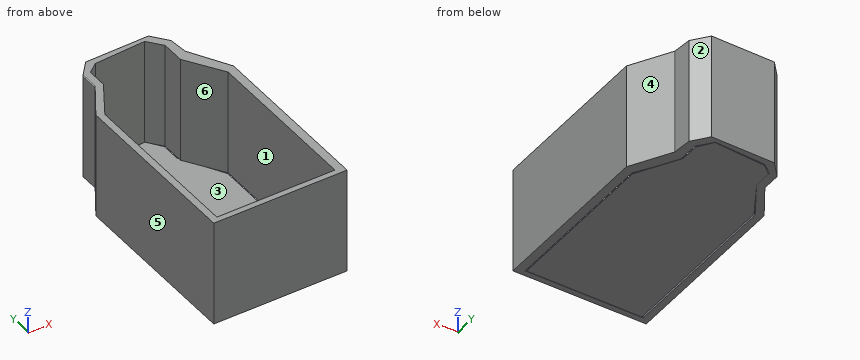
from build123d import *

# Parameters (mm, degrees)
F1_DEPTH = 53.34
F3_DEPTH = 0.254
F4_R     = 0.427399


with BuildPart() as f1:
    # F0 (on Top) → F1 (new body)
    with BuildSketch(Plane.XY):
        Polygon((-29.670693, 53.525094), (-40.17527, 37.058461), (-40.17527, -53.224109), (27.1108, -53.224109), (27.1108, 33.651568), (15.754499, 53.525094), (14.902776, 62.894039), (8.656814, 70.843451), (-23.42473, 70.275635), (-29.670693, 62.894039), align=None)
        Polygon((-25.695989, 63.177943), (-20.585654, 67.152657), (5.249925, 68.572186), (10.928073, 61.474502), (10.928073, 49.834296), (22.85219, 31.380311), (22.85219, -50.385039), (-36.768381, -50.385039), (-36.768381, 35.355017), (-25.695989, 53.241186), align=None, mode=Mode.SUBTRACT)
    extrude(amount=F1_DEPTH)

    # F2 (on Top) → F3 (join)
    with BuildSketch(Plane.XY):
        Polygon((-18.457072, 66.836618), (-20.728331, 66.836618), (-25.554758, 62.578008), (-25.554758, 53.492971), (-35.775427, 35.890706), (-35.775427, -49.84935), (22.425605, -49.84935), (22.425605, 31.064278), (10.501488, 51.789522), (10.501488, 61.442375), (5.391155, 68.540059), align=None)
    extrude(amount=-F3_DEPTH)

    # F4
    f4_edges = [f1.edges().sort_by_distance(p)[0] for p in [
        (-36.768381, 35.355017, 26.67),
        (-29.670693, 58.209566, 53.34),
        (15.754499, 53.525094, 26.67),
    ]]
    fillet(f4_edges, radius=F4_R)


solid = f1.part
Read the model definition and answer for the solid it produces. Units are mm, in the model's axes. Face numbers are marked on the shaded views. A direction names the side the tool comes from. Give positions to 0.01 mm unless a question says otherwise; leave off trailing zeros. Loops run counter-clockwise (first coordinate to the right, second up) from the corner with the lowest first, then second, coordinate; pieces in that order, holes last. Notation, with made-up numbers: (57, 14) -> (113, 14) arc R22 cw to (113, 52) -> close; hole circle Ø11 at (-17.5, -39.5). An arc over 180 degrees is marked (long way). Answer as CSV lines item,"result".
Item 1: Determine the mould class of the marked faces 4, 5 and 6 for opening direction X: +X half, -X half, draft (parallel to the pull), parting line (faces both ways), or undercut.
Returned:
face 4,"+X half"
face 5,"-X half"
face 6,"undercut"
Item 2: Each of these flat-tipped pins is pushed along its axis until it touches: pin 1 (2 mm diameter, centred on x = 4.5, y = 57.5, fed in from +Z); pin 2 (1.5 mm diameter, centred on y = 55.5, z = 6.5, fed in from +X); pin 3 (10 mm diameter, centred on x = 1, z = 5.5, fed in from +Y). Where does it stop, or does it pass through?
Returned:
pin 1,"stops at z = 0"
pin 2,"stops at x = 15.64"
pin 3,"stops at y = 70.8"
Item 3: Find section D-D on y = 48.5. Give the vertices of the cut face in (x, z), plus the area to 3 significant figures.
Returned:
outline,"(-32.88, 0) -> (-28.63, 0) -> (-28.63, 53.34) -> (-32.88, 53.34) -> close; (-28.45, -0.25) -> (12.39, -0.25) -> (12.39, 0) -> (18.63, 0) -> (18.63, 53.34) -> (11.79, 53.34) -> (11.79, 0) -> (-28.45, 0) -> close"
area,"601 mm²"
Item 4: Consider line 1 (X direction, y = -12, z = 26); line 2 (Z direction, x = 13.5, y = 32.5); line 3 (X direction, y = 58.5, z = 13). Determine where each line is inside the solid, lowest interval first. Write a range as [from, to].
Returned:
line 1,"x = [-40.18, -36.77], [22.85, 27.11]"
line 2,"z = [-0.25, 0]"
line 3,"x = [-29.67, -25.7], [10.93, 15.3]"
Item 5: For the marked faces 1, 2 and 3, determine the directions among +Z, -Z, +X, -X, +Y, -Y from which every point of the face is accessible in a straight line to the end or side of a thin tool.
Returned:
face 1,"+Z, -Z"
face 2,"+Z, -Z, +X, +Y"
face 3,"+Z"
Item 6: Find section B-B on x = -11. Give the vertices of the cut face in (y, z), plus the area to 3 significant figures.
Returned:
outline,"(-53.22, 0) -> (-50.39, 0) -> (-50.39, 53.34) -> (-53.22, 53.34) -> close; (-49.85, -0.25) -> (67.37, -0.25) -> (67.37, 0) -> (-49.85, 0) -> close; (67.68, 0) -> (70.5, 0) -> (70.5, 53.34) -> (67.68, 53.34) -> close"
area,"331 mm²"
Item 7: Find section A-A on y = 29.5. Give the vertices of the cut face in (x, z).
Returned:
outline,"(-40.18, 0) -> (-36.77, 0) -> (-36.77, 53.34) -> (-40.18, 53.34) -> close; (-35.78, -0.25) -> (22.43, -0.25) -> (22.43, 0) -> (-35.78, 0) -> close; (22.85, 0) -> (27.11, 0) -> (27.11, 53.34) -> (22.85, 53.34) -> close"
Item 8: Find section C-C on z = 38.5. Give the vertices of the cut face in (x, y), plus the area to 3 significant figures.
Returned:
outline,"(-40.18, -53.22) -> (27.11, -53.22) -> (27.11, 33.65) -> (15.8, 53.44) arc R0.43 cw to (15.75, 53.62) -> (14.9, 62.89) -> (8.66, 70.84) -> (-23.42, 70.28) -> (-29.67, 62.89) -> (-29.67, 53.53) -> (-40.18, 37.06) -> close; hole (-36.77, -50.39) -> (22.85, -50.39) -> (22.85, 31.38) -> (10.93, 49.83) -> (10.93, 61.47) -> (5.25, 68.57) -> (-20.59, 67.15) -> (-25.7, 63.18) -> (-25.7, 53.24) -> (-36.7, 35.46) arc R0.43 ccw to (-36.77, 35.23) -> close"
area,"1,260 mm²"
